from build123d import *

# Parameters (mm, degrees)
SKETCH1_R           = 2.5
BOSS_EXTRUDE3_DEPTH = 5


with BuildPart() as part:
    # Sketch1 → Boss-Extrude3 (new body)
    with BuildSketch(Plane.XY):
        Polygon((4.907477288, 0), (2.453738644, 4.25), (-2.453738644, 4.25), (-4.907477288, 0), (-2.453738644, -4.25), (2.453738644, -4.25), align=None)
        Circle(SKETCH1_R, mode=Mode.SUBTRACT)
    extrude(amount=-BOSS_EXTRUDE3_DEPTH)


solid = part.part
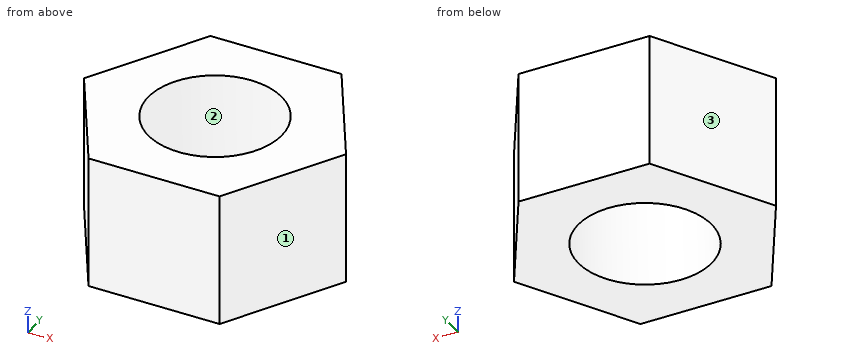
Geometry check sheet. Reference: the model listing, model coordinates, mm. Face numbers are marked on the shaded views. Give positions to 0.01 mm unless a question says otherwise; leave off trailing zeros. Loops run counter-clockwise (first coordinate to the right, second up) from the corner with the lowest first, then second, coordinate; pieces in that order, holes last.
(1) Depth check by flat-ended pin: pin 1 Ø2 at (y, z) = (2, -4) entering from -X; pin 2 Ø1.5 at (y, z) = (-1.5, -2.5) entering from +X. Enter the tip coordinate at first touch or a pass-through.
From the geometry:
pin 1: stops at x = -4.33
pin 2: stops at x = 4.47
(2) Release check for a two-part mould opening along Y. For the marked faces 1, 2 and 3 record: released by +Y, released by -Y, zero draft, split by the parting line, or undercut.
From the geometry:
face 1: released by -Y
face 2: undercut
face 3: released by +Y
(3) Section check D-D on y = -3.25. Record the cut outline in (x, z).
From the geometry:
outline: (-3.03, -5) - (3.03, -5) - (3.03, 0) - (-3.03, 0) - close
(4) Section check B-B on z = -2.05. Record the cut outline in (x, y).
From the geometry:
outline: (-4.91, 0) - (-2.45, -4.25) - (2.45, -4.25) - (4.91, 0) - (2.45, 4.25) - (-2.45, 4.25) - close; hole circle Ø5 at (0, 0)
(5) Section check C-C on x = 0. Record the cut outline in (y, z), then the cut area to 3 significant figures.
From the geometry:
outline: (-4.25, -5) - (-2.5, -5) - (-2.5, 0) - (-4.25, 0) - close; (2.5, -5) - (4.25, -5) - (4.25, 0) - (2.5, 0) - close
area: 17.5 mm2
(6) Section check A-A on x = 1.5. Record the cut outline in (y, z).
From the geometry:
outline: (-4.25, -5) - (-2, -5) - (-2, 0) - (-4.25, 0) - close; (2, -5) - (4.25, -5) - (4.25, 0) - (2, 0) - close
(7) Thickness scan on L1, parallel to Y at x = 0, z = -3.15; L2, parallel to Y at x = 2, z = -2.65; L3, parallel to X at y = -0.5, z = -2. Record the ranges inside material, lowest first.
From the geometry:
L1: y = -4.25 to -2.5, 2.5 to 4.25
L2: y = -4.25 to -1.5, 1.5 to 4.25
L3: x = -4.62 to -2.45, 2.45 to 4.62
